from build123d import *

# Parameters (mm, degrees)
SKETCH1_R           = 2.5
SKETCH1_R_2         = 3.57
BOSS_EXTRUDE1_DEPTH = 1.5


with BuildPart() as part:
    # Sketch1 → Boss-Extrude1 (new body, symmetric)
    with BuildSketch(Plane.XY):
        with BuildLine():
            Line((-60.14, -44), (60.14, -44))
            ThreePointArc((60.14, -44), (62.515878785, -43.015878785), (63.5, -40.64))
            Line((63.5, -40.64), (63.5, 40.64))
            ThreePointArc((63.5, 40.64), (62.515878785, 43.015878785), (60.14, 44))
            Line((60.14, 44), (-60.14, 44))
            ThreePointArc((-60.14, 44), (-62.515878785, 43.015878785), (-63.5, 40.64))
            Line((-63.5, 40.64), (-63.5, -40.64))
            ThreePointArc((-63.5, -40.64), (-62.515878785, -43.015878785), (-60.14, -44))
        make_face()
        with Locations((0, -20)):
            Circle(SKETCH1_R, mode=Mode.SUBTRACT)
        with Locations((10, -20)):
            Circle(SKETCH1_R, mode=Mode.SUBTRACT)
        with Locations((20, -20)):
            Circle(SKETCH1_R, mode=Mode.SUBTRACT)
        with Locations((30, -20)):
            Circle(SKETCH1_R, mode=Mode.SUBTRACT)
        with Locations((40, -20)):
            Circle(SKETCH1_R, mode=Mode.SUBTRACT)
        with Locations((50, -20)):
            Circle(SKETCH1_R, mode=Mode.SUBTRACT)
        with Locations((-10, -20)):
            Circle(SKETCH1_R, mode=Mode.SUBTRACT)
        with Locations((-20, -20)):
            Circle(SKETCH1_R, mode=Mode.SUBTRACT)
        with Locations((-30, -20)):
            Circle(SKETCH1_R, mode=Mode.SUBTRACT)
        with Locations((-40, -20)):
            Circle(SKETCH1_R, mode=Mode.SUBTRACT)
        with Locations((-50, -20)):
            Circle(SKETCH1_R, mode=Mode.SUBTRACT)
        with Locations((-50, -30)):
            Circle(SKETCH1_R, mode=Mode.SUBTRACT)
        with Locations((-40, -30)):
            Circle(SKETCH1_R, mode=Mode.SUBTRACT)
        with Locations((-30, -30)):
            Circle(SKETCH1_R, mode=Mode.SUBTRACT)
        with Locations((-20, -30)):
            Circle(SKETCH1_R, mode=Mode.SUBTRACT)
        with Locations((50, -30)):
            Circle(SKETCH1_R_2, mode=Mode.SUBTRACT)
        with Locations((40, -30)):
            Circle(SKETCH1_R_2, mode=Mode.SUBTRACT)
        with Locations((30, -30)):
            Circle(SKETCH1_R_2, mode=Mode.SUBTRACT)
        with Locations((20, -30)):
            Circle(SKETCH1_R_2, mode=Mode.SUBTRACT)
        with Locations((-50, 0)):
            Circle(SKETCH1_R, mode=Mode.SUBTRACT)
        with Locations((-40, 0)):
            Circle(SKETCH1_R, mode=Mode.SUBTRACT)
        with Locations((-30, 0)):
            Circle(SKETCH1_R, mode=Mode.SUBTRACT)
        with Locations((-20, 0)):
            Circle(SKETCH1_R, mode=Mode.SUBTRACT)
        with Locations((-10, 0)):
            Circle(SKETCH1_R, mode=Mode.SUBTRACT)
        Circle(SKETCH1_R, mode=Mode.SUBTRACT)
        with Locations((10, 0)):
            Circle(SKETCH1_R, mode=Mode.SUBTRACT)
        with Locations((20, 0)):
            Circle(SKETCH1_R_2, mode=Mode.SUBTRACT)
        with Locations((30, 0)):
            Circle(SKETCH1_R_2, mode=Mode.SUBTRACT)
        with Locations((40, 0)):
            Circle(SKETCH1_R_2, mode=Mode.SUBTRACT)
        with Locations((50, 0)):
            Circle(SKETCH1_R_2, mode=Mode.SUBTRACT)
        with Locations((-30, -10)):
            Circle(SKETCH1_R, mode=Mode.SUBTRACT)
        with Locations((-20, -10)):
            Circle(SKETCH1_R, mode=Mode.SUBTRACT)
        with Locations((20, -10)):
            Circle(SKETCH1_R, mode=Mode.SUBTRACT)
        with Locations((30, -10)):
            Circle(SKETCH1_R, mode=Mode.SUBTRACT)
        with Locations((0, -10)):
            Circle(SKETCH1_R, mode=Mode.SUBTRACT)
        with Locations((-15, -15)):
            Circle(SKETCH1_R, mode=Mode.SUBTRACT)
        with Locations((15, -15)):
            Circle(SKETCH1_R, mode=Mode.SUBTRACT)
        with Locations((15, 15)):
            Circle(SKETCH1_R, mode=Mode.SUBTRACT)
        with Locations((-15, 15)):
            Circle(SKETCH1_R, mode=Mode.SUBTRACT)
        with Locations((0, 10)):
            Circle(SKETCH1_R, mode=Mode.SUBTRACT)
        with Locations((30, 10)):
            Circle(SKETCH1_R, mode=Mode.SUBTRACT)
        with Locations((20, 10)):
            Circle(SKETCH1_R, mode=Mode.SUBTRACT)
        with Locations((-20, 10)):
            Circle(SKETCH1_R, mode=Mode.SUBTRACT)
        with Locations((-30, 10)):
            Circle(SKETCH1_R, mode=Mode.SUBTRACT)
        with Locations((20, 30)):
            Circle(SKETCH1_R_2, mode=Mode.SUBTRACT)
        with Locations((30, 30)):
            Circle(SKETCH1_R_2, mode=Mode.SUBTRACT)
        with Locations((40, 30)):
            Circle(SKETCH1_R_2, mode=Mode.SUBTRACT)
        with Locations((50, 30)):
            Circle(SKETCH1_R_2, mode=Mode.SUBTRACT)
        with Locations((-20, 30)):
            Circle(SKETCH1_R, mode=Mode.SUBTRACT)
        with Locations((-30, 30)):
            Circle(SKETCH1_R, mode=Mode.SUBTRACT)
        with Locations((-40, 30)):
            Circle(SKETCH1_R, mode=Mode.SUBTRACT)
        with Locations((-50, 30)):
            Circle(SKETCH1_R, mode=Mode.SUBTRACT)
        with Locations((-50, 20)):
            Circle(SKETCH1_R, mode=Mode.SUBTRACT)
        with Locations((-40, 20)):
            Circle(SKETCH1_R, mode=Mode.SUBTRACT)
        with Locations((-30, 20)):
            Circle(SKETCH1_R, mode=Mode.SUBTRACT)
        with Locations((-20, 20)):
            Circle(SKETCH1_R, mode=Mode.SUBTRACT)
        with Locations((-10, 20)):
            Circle(SKETCH1_R, mode=Mode.SUBTRACT)
        with Locations((50, 20)):
            Circle(SKETCH1_R, mode=Mode.SUBTRACT)
        with Locations((40, 20)):
            Circle(SKETCH1_R, mode=Mode.SUBTRACT)
        with Locations((30, 20)):
            Circle(SKETCH1_R, mode=Mode.SUBTRACT)
        with Locations((20, 20)):
            Circle(SKETCH1_R, mode=Mode.SUBTRACT)
        with Locations((10, 20)):
            Circle(SKETCH1_R, mode=Mode.SUBTRACT)
        with Locations((0, 20)):
            Circle(SKETCH1_R, mode=Mode.SUBTRACT)
        with BuildLine():
            Line((-10, -27.5), (10, -27.5))
            ThreePointArc((10, -27.5), (12.5, -30), (10, -32.5))
            Line((10, -32.5), (-10, -32.5))
            ThreePointArc((-10, -32.5), (-12.5, -30), (-10, -27.5))
        make_face(mode=Mode.SUBTRACT)
        with BuildLine():
            Line((-23.25, -36.52), (-16.75, -36.52))
            ThreePointArc((-16.75, -36.52), (-15.25, -38.02), (-16.75, -39.52))
            Line((-16.75, -39.52), (-23.25, -39.52))
            ThreePointArc((-23.25, -39.52), (-24.75, -38.02), (-23.25, -36.52))
        make_face(mode=Mode.SUBTRACT)
        with BuildLine():
            Line((-3.25, -36.52), (3.25, -36.52))
            ThreePointArc((3.25, -36.52), (4.75, -38.02), (3.25, -39.52))
            Line((3.25, -39.52), (-3.25, -39.52))
            ThreePointArc((-3.25, -39.52), (-4.75, -38.02), (-3.25, -36.52))
        make_face(mode=Mode.SUBTRACT)
        with BuildLine():
            Line((16.75, -36.52), (23.25, -36.52))
            ThreePointArc((23.25, -36.52), (24.75, -38.02), (23.25, -39.52))
            Line((23.25, -39.52), (16.75, -39.52))
            ThreePointArc((16.75, -39.52), (15.25, -38.02), (16.75, -36.52))
        make_face(mode=Mode.SUBTRACT)
        with BuildLine():
            Line((-10, 27.5), (10, 27.5))
            ThreePointArc((10, 27.5), (12.5, 30), (10, 32.5))
            Line((10, 32.5), (-10, 32.5))
            ThreePointArc((-10, 32.5), (-12.5, 30), (-10, 27.5))
        make_face(mode=Mode.SUBTRACT)
        with BuildLine():
            Line((-23.25, 36.52), (-16.75, 36.52))
            ThreePointArc((-16.75, 36.52), (-15.25, 38.02), (-16.75, 39.52))
            Line((-16.75, 39.52), (-23.25, 39.52))
            ThreePointArc((-23.25, 39.52), (-24.75, 38.02), (-23.25, 36.52))
        make_face(mode=Mode.SUBTRACT)
        with BuildLine():
            Line((-3.25, 36.52), (3.25, 36.52))
            ThreePointArc((3.25, 36.52), (4.75, 38.02), (3.25, 39.52))
            Line((3.25, 39.52), (-3.25, 39.52))
            ThreePointArc((-3.25, 39.52), (-4.75, 38.02), (-3.25, 36.52))
        make_face(mode=Mode.SUBTRACT)
        with BuildLine():
            Line((16.75, 36.52), (23.25, 36.52))
            ThreePointArc((23.25, 36.52), (24.75, 38.02), (23.25, 39.52))
            Line((23.25, 39.52), (16.75, 39.52))
            ThreePointArc((16.75, 39.52), (15.25, 38.02), (16.75, 36.52))
        make_face(mode=Mode.SUBTRACT)
    extrude(amount=BOSS_EXTRUDE1_DEPTH, both=True)


solid = part.part
Here's how the part is built. I have some questions about the finished solid (model axes, mm). A direction names the side the tool comes from. Coordinates: 2 decimals unless noted, no trailing zeros. Loops run counter-clockwise (first coordinate to the right, second up) from the corner with the lowest first, then second, coordinate; pieces in that order, holes last.
1. I need wall thicknesses on L1, parallel to Y at x = -15, z = 0.25; L2, parallel to Y at x = 10, z = -0.75; L3, parallel to Y at x = -7, z = 1.05. Which ranges of each line are inside material? Lowest first, please.
2. Imagine slicing it at A-A, the plane y = -10. Please give me the cut outline in (x, z), and give its area (3 significant figures).
3. For faces 1 (the flat face through (1, 44, 0)), 2 (the flat face through (0, 39.52, 0)), which set-ups out of +Z, -Z, +X, -X, +Y, -Y let a thin tool reach every point of the face, with its end or its side?
4. Imagine slicing it at B-B, the plane x = 0. Count the separate pieces of the cut face and the enclosed holes in it, and give its area (3 significant figures).
Taken from the geometry:
1. L1: y = -44 to -17.5, -12.5 to 12.5, 17.5 to 44
1. L2: y = -44 to -32.5, -27.5 to -22.5, -17.5 to -2.5, 2.5 to 17.5, 22.5 to 27.5, 32.5 to 44
1. L3: y = -44 to -32.5, -27.5 to 27.5, 32.5 to 44
2. outline: (-63.5, -1.5) - (-32.5, -1.5) - (-32.5, 1.5) - (-63.5, 1.5) - close; (-27.5, -1.5) - (-22.5, -1.5) - (-22.5, 1.5) - (-27.5, 1.5) - close; (-17.5, -1.5) - (-2.5, -1.5) - (-2.5, 1.5) - (-17.5, 1.5) - close; (2.5, -1.5) - (17.5, -1.5) - (17.5, 1.5) - (2.5, 1.5) - close; (22.5, -1.5) - (27.5, -1.5) - (27.5, 1.5) - (22.5, 1.5) - close; (32.5, -1.5) - (63.5, -1.5) - (63.5, 1.5) - (32.5, 1.5) - close
2. area: 306 mm2
3. face 1: +Z, -Z, +X, -X, +Y
3. face 2: +Z, -Z
4. separate pieces: 10
4. enclosed holes: 0
4. area: 141 mm2
